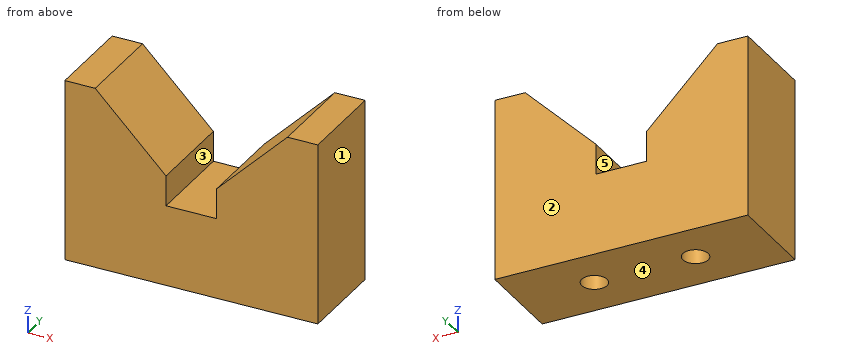
from build123d import *

# Parameters (mm, degrees)
F1_DEPTH = 4.5
F3_D     = 2.5
F3_DEPTH = 7
F3_TIP   = 0.7510757738


with BuildPart() as f1:
    # F0 (on Front) → F1 (new body, symmetric)
    with BuildSketch(Plane.XZ):
        Polygon((0, 8), (0, 0), (12.5, 0), (12.5, 18), (9.5, 18), (2.5, 11), (2.5, 8), align=None)
    extrude(amount=F1_DEPTH, both=True)

    # F3
    with Locations(Plane(origin=(0, 0, 0), x_dir=(1, 0, 0), z_dir=(0, 0, -1))):
        with Locations((5, 0)):
            Hole(F3_D / 2, depth=F3_DEPTH)
            with Locations((0, 0, -(F3_DEPTH + F3_TIP / 2))):  # 118° drill point
                Cone(0, F3_D / 2, F3_TIP, mode=Mode.SUBTRACT)

    # F4: F1 across plane


with BuildPart() as f1_1:
    add(f1.part)
    add(f1.part.mirror(Plane.YZ))


solid = f1_1.part
Read the model definition and answer for the solid it produces. Units are mm, in the model's axes. Face numbers are marked on the shaded views. A direction names the side the tool comes from. Round coordinates to 2 decimals unless told otherwise and drop trailing zeros. Loops run counter-clockwise (first coordinate to the right, second up) from the corner with the lowest first, then second, coordinate; pieces in that order, holes last.
Q1. Which of the six approach directions +Z, -Z, +X, -X, +Y, -Y give full straight-line access (tool end or side, diameter ignored) to the marked faces 4 and 5?
Q2. Consider probe 1 along Y at (x, z) = (5, 2.5); probe 2 along X at (y, z) = (-0.75, 12.25); probe 3 along Z at (x, y) = (-1.5, 0.75). Determine where each line is inside the solid, lowest interval first.
Q3. Section B-B on z = 6.25 is taken. Write down the section's boundary in (x, y), and give its area (3 significant figures).
Q4. Section C-C on y = 1.75 is taken. Write down the section's boundary in (x, z), and give its area (3 significant figures).
Q5. Determine the mould class of the marked faces 1, 2 and 3 for opening direction X: released by +X, released by -X, zero draft, split by the parting line, or undercut.
Q6. Each of these flat-tipped pins is pushed along its axis until it touches: pin 1 (1.5 mm diameter, centred on x = 1, y = 1, fed in from +Z); pin 2 (2 mm diameter, centred on x = -5, y = 0, fed in from -Z). Where does it stop, or does it pass through?
Q7. Section A-A on z = 13 is taken. Write down the section's boundary in (x, y), and give its area (3 significant figures).
Q8. Section D-D on z = 9.5 is taken. Write down the section's boundary in (x, y).
Output:
1. face 4: -Z, +X, -X, +Y, -Y
1. face 5: +Z, +Y, -Y
2. probe 1: y = -4.5 to -1.25, 1.25 to 4.5
2. probe 2: x = -12.5 to -3.75, 3.75 to 12.5
2. probe 3: z = 0 to 8
3. outline: (-12.5, -4.5) - (12.5, -4.5) - (12.5, 4.5) - (-12.5, 4.5) - close; hole circle Ø2.5 at (-5, 0); hole circle Ø2.5 at (5, 0)
3. area: 215 mm2
4. outline: (-12.5, 0) - (12.5, 0) - (12.5, 18) - (9.5, 18) - (2.5, 11) - (2.5, 8) - (-2.5, 8) - (-2.5, 11) - (-9.5, 18) - (-12.5, 18) - close
4. area: 351 mm2
5. face 1: released by +X
5. face 2: zero draft
5. face 3: undercut
6. pin 1: stops at z = 8
6. pin 2: stops at z = 7.15
7. outline: (-12.5, -4.5) - (-4.5, -4.5) - (-4.5, 4.5) - (-12.5, 4.5) - close; (4.5, -4.5) - (12.5, -4.5) - (12.5, 4.5) - (4.5, 4.5) - close
7. area: 144 mm2
8. outline: (-12.5, -4.5) - (-2.5, -4.5) - (-2.5, 4.5) - (-12.5, 4.5) - close; (2.5, -4.5) - (12.5, -4.5) - (12.5, 4.5) - (2.5, 4.5) - close
